Autodesk Fusion 360 part; units mm, degrees
sketch "草图1" plane through (0, 0, 0) normal (0, 0, 1) x (1, 0, 0)
  line L0 (57.5, -10) -> (25, -10)
  line L1 (25, -10) -> (25, 0)
  line L2 (25, 0) -> (150, 0)
  line L3 (57.5, -5) -> (57.5, -10)
  line L4 (87.5, 0) -> (117.5, 0)
  arc A0 (137.5, -5) -> (137.5, 0) centre (137.5, -2.5) ccw
  line L5 (150, 30) -> (145, 30)
  arc A1 (37.5, 0) -> (37.5, -5) centre (37.5, -2.5) ccw
  line L6 (150, -10) -> (117.5, -10)
  line L7 (140, 110) -> (140, 60)
  line L8 (150, 120) -> (25, 120)
  line L9 (150, 90) -> (145, 90)
  line L10 (150, 90) -> (150, 120)
  line L11 (87.5, 0) -> (87.5, 120) construction
  line L12 (117.5, -5) -> (117.5, -10)
  line L13 (145, 30) -> (145, 10)
  arc A2 (140, 10) -> (145, 10) centre (142.5, 10) ccw
  line L14 (150, 0) -> (150, 30)
  line L15 (150, 0) -> (150, -10)
  line L16 (137.5, -5) -> (117.5, -5)
  line L17 (140, 10) -> (140, 60)
  line L18 (145, 90) -> (145, 110)
  arc A3 (145, 110) -> (140, 110) centre (142.5, 110) ccw
  line L19 (57.5, -5) -> (37.5, -5)
  line L20 (25, 0) -> (150, 0)
  line L21 (25, 120) -> (25, 0)
  dimension "d1" = 120
  dimension "d2" = 125
  dimension "d3" = 100
  dimension "d4" = 20
  dimension "d5" = 20
  dimension "d6" = 5
  dimension "d7" = 5
  dimension "d8" = 2.5
  dimension "d9" = 2.5
  dimension "d10" = 10
extrude "拉伸1" add sketch "草图1" along normal blind 10 makes body 1
sketch "草图2" plane through (0, 0, 0) normal (0, 0, -1) x (1, 0, 0)
  line L0 (150, -120) -> (150, -90)
  line L1 (150, -90) -> (145, -90)
  line L2 (145, -90) -> (145, -110)
  arc A0 (140, -110) -> (145, -110) centre (142.5, -110) ccw
  line L3 (140, -110) -> (140, -10)
  arc A1 (145, -10) -> (140, -10) centre (142.5, -10) ccw
  line L4 (145, -10) -> (145, -30)
  line L5 (145, -30) -> (150, -30)
  line L6 (150, -30) -> (150, 10)
  line L7 (150, 10) -> (117.5, 10)
  line L8 (117.5, 10) -> (117.5, 5)
  line L9 (117.5, 5) -> (137.5, 5)
  arc A2 (137.5, 0) -> (137.5, 5) centre (137.5, 2.5) ccw
  line L10 (137.5, 0) -> (37.5, 0)
  arc A3 (37.5, 5) -> (37.5, 0) centre (37.5, 2.5) ccw
  line L11 (37.5, 5) -> (57.5, 5)
  line L12 (57.5, 5) -> (57.5, 10)
  line L13 (57.5, 10) -> (25, 10)
  line L14 (25, 10) -> (25, -120)
  line L15 (25, -120) -> (150, -120)
  line L16 (45.5, -10.5) -> (119.5, -10.5)
  line L17 (129.5, -20.5) -> (129.5, -99.5)
  line L18 (119.5, -109.5) -> (45.5, -109.5)
  line L19 (35.5, -99.5) -> (35.5, -20.5)
  arc A4 (45.5, -10.5) -> (35.5, -20.5) centre (45.5, -20.5) ccw
  arc A5 (129.5, -20.5) -> (119.5, -10.5) centre (119.5, -20.5) ccw
  arc A6 (119.5, -109.5) -> (129.5, -99.5) centre (119.5, -99.5) ccw
  arc A7 (35.5, -99.5) -> (45.5, -109.5) centre (45.5, -99.5) ccw
  point P0 (35.5, -10.5)
  point P1 (129.5, -10.5)
  point P2 (35.5, -109.5)
  dimension "d13" = 94
  dimension "d14" = 99
  dimension "d15" = 10.5
  dimension "d16" = 10.5
  dimension "d17" = 10.5
  dimension "d18" = 10.5
  dimension "d19" = 10
  dimension "d20" = 10
  dimension "d21" = 10
  dimension "d22" = 10
extrude "拉伸2" add sketch "草图2" along normal blind 5 contours L16 L17 L18 L19 A4 A5 A6 A7 bodies 1
sketch "草图3" plane through (0, 0, 0) normal (0, 0, -1) x (1, 0, 0)
  line L0 (45.5, -10.5) -> (119.5, -10.5)
  arc A0 (129.5, -20.5) -> (119.5, -10.5) centre (119.5, -20.5) ccw
  line L1 (129.5, -20.5) -> (129.5, -99.5)
  arc A1 (119.5, -109.5) -> (129.5, -99.5) centre (119.5, -99.5) ccw
  line L2 (119.5, -109.5) -> (45.5, -109.5)
  arc A2 (35.5, -99.5) -> (45.5, -109.5) centre (45.5, -99.5) ccw
  line L3 (35.5, -99.5) -> (35.5, -20.5)
  arc A3 (45.5, -10.5) -> (35.5, -20.5) centre (45.5, -20.5) ccw
  line L4 (150, -120) -> (150, -90)
  line L5 (150, -90) -> (145, -90)
  line L6 (145, -90) -> (145, -110)
  arc A4 (140, -110) -> (145, -110) centre (142.5, -110) ccw
  line L7 (140, -110) -> (140, -10)
  arc A5 (145, -10) -> (140, -10) centre (142.5, -10) ccw
  line L8 (145, -10) -> (145, -30)
  line L9 (145, -30) -> (150, -30)
  line L10 (150, -30) -> (150, 10)
  line L11 (150, 10) -> (117.5, 10)
  line L12 (117.5, 10) -> (117.5, 5)
  line L13 (117.5, 5) -> (137.5, 5)
  arc A6 (137.5, 0) -> (137.5, 5) centre (137.5, 2.5) ccw
  line L14 (137.5, 0) -> (37.5, 0)
  arc A7 (37.5, 5) -> (37.5, 0) centre (37.5, 2.5) ccw
  line L15 (37.5, 5) -> (57.5, 5)
  line L16 (57.5, 5) -> (57.5, 10)
  line L17 (57.5, 10) -> (25, 10)
  line L18 (25, 10) -> (25, -120)
  line L19 (25, -120) -> (150, -120)
  line L20 (30.5, -5.5) -> (44.5, -5.5)
  line L21 (44.5, -5.5) -> (44.5, -7.5)
  line L22 (44.5, -7.5) -> (32.5, -7.5)
  line L23 (30.5, -7.5) -> (30.5, -5.5)
  line L24 (30.5, -5.5) -> (33.5, -5.5)
  line L25 (32.5, -7.5) -> (32.5, -19.5)
  line L26 (32.5, -19.5) -> (30.5, -19.5)
  line L27 (30.5, -19.5) -> (30.5, -5.5)
  line L28 (120.5, -5.5) -> (134.5, -5.5)
  line L29 (134.5, -5.5) -> (134.5, -8.5)
  line L30 (132.5, -7.5) -> (120.5, -7.5)
  line L31 (120.5, -7.5) -> (120.5, -5.5)
  line L32 (134.5, -5.5) -> (131.5, -5.5)
  line L33 (132.5, -7.5) -> (132.5, -19.5)
  line L34 (132.5, -19.5) -> (134.5, -19.5)
  line L35 (134.5, -19.5) -> (134.5, -5.5)
  line L36 (30.5, -100.5) -> (32.5, -100.5)
  line L37 (32.5, -100.5) -> (32.5, -112.5)
  line L38 (33.5, -114.5) -> (30.5, -114.5)
  line L39 (30.5, -114.5) -> (30.5, -100.5)
  line L40 (30.5, -114.5) -> (44.5, -114.5)
  line L41 (44.5, -114.5) -> (44.5, -112.5)
  line L42 (44.5, -112.5) -> (32.5, -112.5)
  line L43 (30.5, -111.5) -> (30.5, -114.5)
  line L44 (120.5, -112.5) -> (132.5, -112.5)
  line L45 (134.5, -112.5) -> (134.5, -114.5)
  line L46 (134.5, -114.5) -> (120.5, -114.5)
  line L47 (120.5, -114.5) -> (120.5, -112.5)
  line L48 (134.5, -114.5) -> (131.5, -114.5)
  line L49 (132.5, -112.5) -> (132.5, -100.5)
  line L50 (132.5, -100.5) -> (134.5, -100.5)
  line L51 (134.5, -100.5) -> (134.5, -114.5)
  dimension "d28" = 14
  dimension "d29" = 5.5
  dimension "d30" = 5.5
  dimension "d31" = 14
  dimension "d32" = 2
  dimension "d34" = 14
  dimension "d35" = 5.5
  dimension "d36" = 5.5
  dimension "d37" = 2
  dimension "d38" = 14
  dimension "d39" = 14
  dimension "d41" = 5.5
  dimension "d42" = 5.5
  dimension "d43" = 14
  dimension "d44" = 2
  dimension "d45" = 14
  dimension "d46" = 5.5
  dimension "d47" = 5.5
  dimension "d107" = 2
  dimension "d108" = 14
  dimension "d109" = 2
  dimension "d110" = 2
  dimension "d111" = 2
  dimension "d112" = 2
extrude "拉伸3" add sketch "草图3" along normal blind 8 contours L20 L21 L22 L23 L24 L25 L26 L27 | L28 L29 L30 L31 L32 L33 L34 L35 | L36 L37 L38 L39 L40 L41 L42 L43 | L44 L45 L46 L47 L48 L49 L50 L51 bodies 1
sketch "草图4" plane through (0, 0, 10) normal (0, 0, 1) x (-1, 0, 0)
  line L0 (-150, -90) -> (-150, -120)
  line L1 (-150, -120) -> (-25, -120)
  line L2 (-25, -120) -> (-25, 10)
  line L3 (-25, 10) -> (-57.5, 10)
  line L4 (-57.5, 10) -> (-57.5, 5)
  line L5 (-57.5, 5) -> (-37.5, 5)
  arc A0 (-37.5, 0) -> (-37.5, 5) centre (-37.5, 2.5) ccw
  line L6 (-37.5, 0) -> (-137.5, 0)
  arc A1 (-137.5, 5) -> (-137.5, 0) centre (-137.5, 2.5) ccw
  line L7 (-137.5, 5) -> (-117.5, 5)
  line L8 (-117.5, 5) -> (-117.5, 10)
  line L9 (-117.5, 10) -> (-150, 10)
  line L10 (-150, 10) -> (-150, -30)
  line L11 (-150, -30) -> (-145, -30)
  line L12 (-145, -30) -> (-145, -10)
  arc A2 (-140, -10) -> (-145, -10) centre (-142.5, -10) ccw
  line L13 (-140, -10) -> (-140, -110)
  arc A3 (-145, -110) -> (-140, -110) centre (-142.5, -110) ccw
  line L14 (-145, -110) -> (-145, -90)
  line L15 (-145, -90) -> (-150, -90)
  line L16 (-40, -105) -> (-85, -105)
  line L17 (-85, -105) -> (-85, -72)
  line L18 (-85, -72) -> (-40, -72)
  line L19 (-40, -72) -> (-40, -105)
  dimension "d50" = 45
  dimension "d51" = 33
  dimension "d52" = 15
  dimension "d53" = 15
extrude "拉伸4" cut sketch "草图4" against normal blind 5 contours L16 L17 L18 L19 bodies 1
fillet "圆角1" radius 5 1 edges at (40, 88.5, 5) on bodies 1
fillet "圆角2" radius 5 1 edges at (85, 88.5, 5) on bodies 1
sketch "草图5" plane through (0, 0, 10) normal (0, 0, 1) x (-1, 0, 0)
  line L0 (-85, -105) -> (-85, -72)
  line L1 (-85, -72) -> (-40, -72)
  line L2 (-40, -72) -> (-40, -105)
  line L3 (-40, -105) -> (-85, -105)
  line L4 (-150, -90) -> (-150, -120)
  line L5 (-150, -120) -> (-25, -120)
  line L6 (-25, -120) -> (-25, 10)
  line L7 (-25, 10) -> (-57.5, 10)
  line L8 (-57.5, 10) -> (-57.5, 5)
  line L9 (-57.5, 5) -> (-37.5, 5)
  arc A0 (-37.5, 0) -> (-37.5, 5) centre (-37.5, 2.5) ccw
  line L10 (-37.5, 0) -> (-137.5, 0)
  arc A1 (-137.5, 5) -> (-137.5, 0) centre (-137.5, 2.5) ccw
  line L11 (-137.5, 5) -> (-117.5, 5)
  line L12 (-117.5, 5) -> (-117.5, 10)
  line L13 (-117.5, 10) -> (-150, 10)
  line L14 (-150, 10) -> (-150, -30)
  line L15 (-150, -30) -> (-145, -30)
  line L16 (-145, -30) -> (-145, -10)
  arc A2 (-140, -10) -> (-145, -10) centre (-142.5, -10) ccw
  line L17 (-140, -10) -> (-140, -110)
  arc A3 (-145, -110) -> (-140, -110) centre (-142.5, -110) ccw
  line L18 (-145, -110) -> (-145, -90)
  line L19 (-145, -90) -> (-150, -90)
  line L20 (-79, -69) -> (-130, -69)
  line L21 (-130, -69) -> (-130, -8)
  line L22 (-130, -8) -> (-79, -8)
  line L23 (-79, -8) -> (-79, -69)
  dimension "d60" = 10
  dimension "d61" = 8
  dimension "d113" = 61
  dimension "d114" = 51
sketch "草图12" plane through (0, 0, 5) normal (0, 0, 1) x (-1, 0, 0)
  line L0 (-80, -72) -> (-80, -105)
  line L1 (-80, -105) -> (-45, -105)
  line L2 (-45, -105) -> (-45, -72)
  line L3 (-45, -72) -> (-80, -72)
  line L4 (-85, -72) -> (-40, -72)
  line L5 (-48, -95.6) -> (-78, -95.6)
  line L6 (-78, -95.6) -> (-78, -77)
  line L7 (-78, -77) -> (-48, -77)
  line L8 (-48, -77) -> (-48, -95.6)
  dimension "d92" = 30
  dimension "d93" = 18.6
  dimension "d94" = 5
  dimension "d95" = 2
extrude "拉伸13" cut sketch "草图12" against normal blind 11 contours L5 L6 L7 L8 bodies 1
copy_body "实体->零部件2" bodies 1 removing the originals makes body 2 in component "Component'"
extrude "拉伸1'" cut sketch "草图5" against normal blind 5 contours L20 L21 L22 L23 bodies 2 in component "Component'"
component "Component'" placed x (1, 0, 0) y (0, 1, 0) z (0, 0, 1) at (0, 0, 0)
Design review of the part built by this model. Coordinates are the model's own, in mm. A direction names the side the tool comes from. Give positions to 0.01 mm unless a question says otherwise; leave off trailing zeros. Loops run counter-clockwise (first coordinate to the right, second up) from the corner with the lowest first, then second, coordinate; pieces in that order, holes last. Notation, with made-up numbers: M 76.5,-26.75 L 95.5,-26.75 A20 cw 95.5,5.25 Z; hole C 87.5,-31.75 d4. An arc over 180 degrees is marked long. Return JSON: item names as keys, results as strings. Group by question number.
Item 1: For probe 1 along Y at (x, z) = (76.5, -1.5); probe 2 along X at (y, z) = (101, 7); probe 3 along Y at (x, z) = (34.5, -6.5), list the stretches that pass through material, from the lowest coordinate up.
Item 2: We need section C-C (x = 73). Give the boundary of the cut face in (y, z), and give its area (3 significant figures).
Item 3: Mouldability with a two-part tool opening along Y and no side actions: class faces 1 (the flat face through (41, -10, 5)), 2 (the flat face through (130, 39, 8)), 3 (the flat face through (131, 7, -8)) as released by +Y, released by -Y, zero draft, split by the parting line, or undercut.
Item 4: We need section B-B (x = 52). Give the boundary of the cut face in (y, z).
Item 5: We need section A-A (y = -2.5). Give the boundary of the cut face in (x, z).
Item 6: We need section D-D (y = 93.5). Give the number of separate pieces and of enclosed holes in the cut face, and give its area (3 significant figures).
Item 7: Tool access review of faces 4 (the flat face through (32.5, 13, -4)), 5 (the flat face through (48, 86, 0)), 6 (the flat face through (63, 72, 8)): name each direction out of +Z, -Z, +X, -X, +Y, -Y from which nothing blocks a thin tool from reaching the whole face with its end or side.
Item 8: Insertion check: pin 1 Ø0.6 at (x, z) = (31.5, -2) entering from -Y; pin 2 Ø4 at (y, z) = (106.5, -3) entering from -X; pin 3 Ø5.5 at (y, z) = (62, -3.5) entering from -X. Each pin has a flat end and moves straight along its axis. Give the tip position at first contact, or say it passes through.
Output:
{
 "1": {"probe 1": "y = 10.5 to 77, 95.6 to 109.5", "probe 2": "x = 25 to 41, 84 to 140, 145 to 150", "probe 3": "y = 5.5 to 7.5, 112.5 to 114.5"},
 "2": {"outline": "M 0,0 L 10.5,0 L 10.5,-5 L 77,-5 L 77,5 L 72,5 L 72,10 L 0,10 Z; M 95.6,-5 L 109.5,-5 L 109.5,0 L 120,0 L 120,10 L 105,10 L 105,5 L 95.6,5 Z", "area": "1,340 mm^2"},
 "3": {"face 1": "released by -Y", "face 2": "undercut", "face 3": "zero draft"},
 "4": {"outline": "M -10,0 L -5,0 L -5,10 L -10,10 Z; M 0,0 L 10.5,0 L 10.5,-5 L 77,-5 L 77,5 L 72,5 L 72,10 L 0,10 Z; M 95.6,-5 L 109.5,-5 L 109.5,0 L 120,0 L 120,10 L 105,10 L 105,5 L 95.6,5 Z"},
 "5": {"outline": "M 25,0 L 35,0 L 35,10 L 25,10 Z; M 140,0 L 150,0 L 150,10 L 140,10 Z"},
 "6": {"separate pieces": "3", "enclosed holes": "0", "area": "1,160 mm^2"},
 "7": {"face 4": "-Z", "face 5": "+Z, -Z", "face 6": "+Z"},
 "8": {"pin 1": "stops at y = 5.5", "pin 2": "stops at x = 30.5", "pin 3": "stops at x = 35.5"}
}
